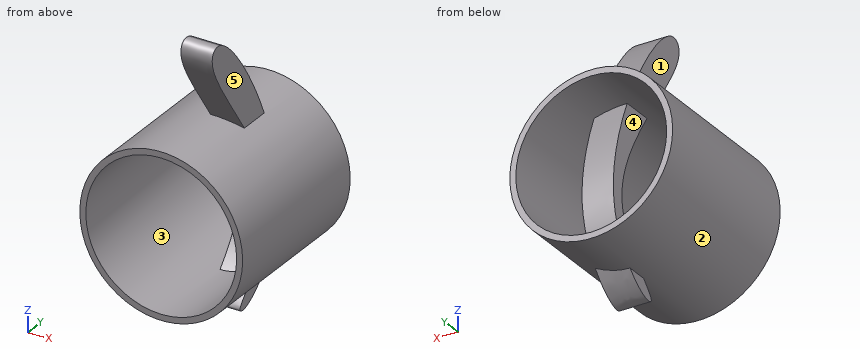
```python
from build123d import *

# Parameters (mm, degrees)
F0_R     = 25
F1_DEPTH = 52.483310923
F4_R     = 23.1594972358
F5_DEPTH = 56.222954765
F7_DEPTH = 9.6091050655


# Not quite as in the source:
# - the program builds the solid bodies; features that only make, move or delete a surface that nothing else refers to are left out


with BuildPart() as f1:
    # F0 (on Front) → F1 (new body)
    with BuildSketch(Plane.XZ):
        Circle(F0_R)
    extrude(amount=-F1_DEPTH)

    # F4 (on face) → F5 (cut)
    with BuildSketch(Plane(origin=(0, 52.483310923, 0), x_dir=(-1, 0, 0), z_dir=(0, 1, 0))):
        Circle(F4_R)
    extrude(amount=-F5_DEPTH, mode=Mode.SUBTRACT)

    # F6 (on Right) → F7 (join)
    with BuildSketch(Plane.YZ):
        with BuildLine():
            add(Edge.make_bspline(
                [(13.5661605746, 52.984289825), (22.7453749365, 49.8663088316), (56.6867603684, -7.723565307), (26.9795580338, -32.0941370462), (20.0288116996, -29.0080395676), (56.4506404561, -5.9541746073), (3.4222546759, 46.2227244929), (10.8831347215, 53.8956557965), (13.5661605746, 52.984289825)],
                knots=[0, 0, 0, 0, 0.2662310005, 0.4435228486, 0.4925757944, 0.6637410127, 0.9221823754, 1, 1, 1, 1], degree=3))
        make_face()
    extrude(amount=F7_DEPTH)


solid = f1.part
```
Verification items for the finished model (mm, model axes). Face numbers are marked on the shaded views. A direction names the side the tool comes from. Coordinates: 2 decimals unless noted, no trailing zeros. Loops run counter-clockwise (first coordinate to the right, second up) from the corner with the lowest first, then second, coordinate; pieces in that order, holes last. Notation, with made-up numbers: (68, -20) -> (102, -20) arc R12 cw to (102, 1) -> close; hole circle Ø8 at (76.25, -25). An arc over 180 degrees is marked (long way). Answer in a Markdown table with one row per item.
1) Scan lines: line 1 along X through (y, z) = (19, 42); line 2 along X through (y, z) = (29, 19); line 3 along Z through (x, y) = (13, 46.5). Record each from-to range of solid material in increasing order. Write a range as from..to.
The answers:
| item | result |
|---|---|
| line 1 | x = 0..9.61 |
| line 2 | x = -16.25..-13.24, 0..9.61, 13.24..16.25 |
| line 3 | z = -21.35..-19.17, 19.17..21.35 |
2) Draft check along X on the marked faces 1, 2 and 3. Enter one of: released by +X, released by -X, zero draft, split by the parting line, or undercut.
The answers:
| item | result |
|---|---|
| face 1 | released by -X |
| face 2 | split by the parting line |
| face 3 | undercut |
3) Access from +Z, -Z, +X, -X, +Y, -Y to the whole of each face (thin tool, end or side, straight path). Record for the marked faces 4 and 5.
The answers:
| item | result |
|---|---|
| face 4 | +Y, -Y |
| face 5 | +Z, +X, +Y, -Y |
4) Section check C-C (z = 12). Give the number of separate pieces and of enclosed holes in the cut face, and give its area (3 significant figures).
The answers:
| item | result |
|---|---|
| separate pieces | 3 |
| enclosed holes | 0 |
| area | 290 mm2 |
5) Section check B-B (y = 7.5). Record the cut outline in (x, z).
The answers:
| item | result |
|---|---|
| outline | circle Ø50 at (0, 0); hole circle Ø46.32 at (0, 0) |
6) Section check A-A (x = 12). Record the cut outline in (y, z).
The answers:
| item | result |
|---|---|
| outline | (0, -21.93) -> (52.48, -21.93) -> (52.48, -19.81) -> (0, -19.81) -> close; (0, 19.81) -> (52.48, 19.81) -> (52.48, 21.93) -> (0, 21.93) -> close |
7) Depth check by flat-ended pin: P1, Ø1, axis at y = 8, z = -3.5, coming from the +X side; P2, Ø2, axis at x = -7, y = 29, coming from the -Z side; P3, Ø20.5, axis at y = 20, z = 35, coming from the +X side; P4, Ø1.5, axis at x = -1, z = 28, coming from the -Y side. Enter the tip coordinate at first touch or a pass-through.
The answers:
| item | result |
|---|---|
| P1 | stops at x = 24.82 |
| P2 | stops at z = -24.27 |
| P3 | stops at x = 9.61 |
| P4 | passes through |
8) Section check D-D (x = -5.5). Record the cut outline in (y, z), and give its area (3 significant figures).
The answers:
| item | result |
|---|---|
| outline | (0, -24.39) -> (52.48, -24.39) -> (52.48, -22.5) -> (0, -22.5) -> close; (0, 22.5) -> (52.48, 22.5) -> (52.48, 24.39) -> (0, 24.39) -> close |
| area | 198 mm2 |
